Autodesk Inventor part; units mm, degrees
ref_plane "YZ Plane" through (0, 0, 0) normal (1, 0, 0) x (0, 1, 0)
ref_plane "XZ Plane" through (0, 0, 0) normal (0, 1, 0) x (-1, 0, 0)
ref_plane "XY Plane" through (0, 0, 0) normal (0, 0, 1) x (1, 0, 0)
sketch "Sketch1" plane through (0, 0, 0) normal (0, 0, 1) x (1, 0, 0)
  line L0 (0, 0) -> (25.4, 0)
  line L1 (25.4, 0) -> (25.4, 25.4)
  line L2 (25.4, 25.4) -> (0, 25.4)
  line L3 (0, 25.4) -> (0, 0)
  line L4 (3.175, 22.225) -> (22.225, 22.225)
  line L5 (22.225, 22.225) -> (22.225, 3.175)
  line L6 (22.225, 3.175) -> (3.175, 3.175)
  line L7 (3.175, 3.175) -> (3.175, 22.225)
  dimension "d0" = 25.4
  dimension "d1" = 25.4
  dimension "d2" = 3.175
extrude "Extrusion1" add sketch "Sketch1" against normal blind 666.75
sketch "Sketch2" plane through (0, 25.4, 0) normal (0, 1, 0) x (1, 0, 0)
  line L0 (25.4, 666.75) -> (0, 666.75)
  line L1 (25.4, 0) -> (0, 0)
  point P0 (12.7, 12.7)
  point P1 (12.7, 38.1)
  point P2 (12.7, 654.05)
  point P3 (12.7, 628.65)
  dimension "d5" = 12.7
  dimension "d6" = 25.4
  dimension "d7" = 25.4
  dimension "d8" = 12.7
hole "Hole1" at (12.7, 25.4, -12.7) at (12.7, 25.4, -38.1) at (12.7, 25.4, -654.05) at (12.7, 25.4, -628.65) direction (0, -1, 0) diameter 6.35 depth 25.4 tip angle 118
properties part number "12 inch middle piece"
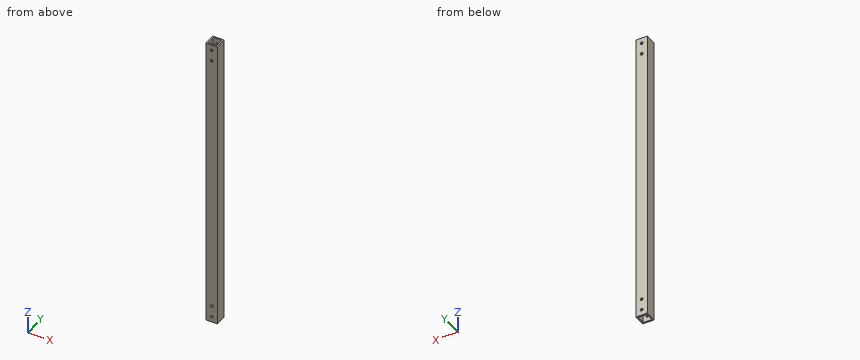
Input: part model. Units: mm. Frame: model coordinates. Coordinates: 2 decimals unless noted, no trailing zeros. Loops run counter-clockwise (first coordinate to the right, second up) from the corner with the lowest first, then second, coordinate; pieces in that order, holes last.
(1) Material intervals for probe 1 along Z at (x, y) = (12.7, 24.25) (3 decimals); probe 2 along X at (y, z) = (23.3, -628.65) (3 decimals); probe 3 along X at (y, z) = (9.5, -490) (3 decimals), sorted ascending.
(2) Section B-B on y = 14.75. Return the cut outline in (x, z) (3 decimals), then the cut area to 3 significant figures.
(3) Section A-A on z = -564.5. Return the cut outline in (x, y) (3 decimals), then the cut area to 3 significant figures.
Data:
1. probe 1: z = -666.75 to -657.225, -650.875 to -631.825, -625.475 to -41.275, -34.925 to -15.875, -9.525 to 0
1. probe 2: x = 0 to 9.525, 15.875 to 25.4
1. probe 3: x = 0 to 3.175, 22.225 to 25.4
2. outline: (0, -666.75) - (3.175, -666.75) - (3.175, 0) - (0, 0) - close; (22.225, -666.75) - (25.4, -666.75) - (25.4, 0) - (22.225, 0) - close
2. area: 4,230 mm2
3. outline: (0, 0) - (25.4, 0) - (25.4, 25.4) - (0, 25.4) - close; hole (3.175, 3.175) - (22.225, 3.175) - (22.225, 22.225) - (3.175, 22.225) - close
3. area: 282 mm2
